Autodesk Inventor part; units mm, degrees
ref_plane "YZ Plane" through (0, 0, 0) normal (1, 0, 0) x (0, 1, 0)
ref_plane "XZ Plane" through (0, 0, 0) normal (0, 1, 0) x (-1, 0, 0)
ref_plane "XY Plane" through (0, 0, 0) normal (0, 0, 1) x (1, 0, 0)
sketch "Esboço1" plane through (0, 0, 0) normal (0, 0, 1) x (1, 0, 0)
  line L0 (-33, -50) -> (-33, 950)
  line L1 (47, -50) -> (47, 950)
  line L2 (-73, -89.8276) -> (47, -89.8276)
  line L3 (47, -9.8276) -> (-73, -9.8276)
  line L4 (-73, -9.8276) -> (-73, -89.8276)
  line L5 (47, -89.8276) -> (47, -9.8276)
  point P0 (0, 0)
  dimension "d0" = 120
  dimension "d1" = 120
  dimension "d2" = 80
extrude "Extrusão1" add sketch "Esboço1" along normal blind 9.52
sketch "Esboço11" plane through (0, 0, 9.52) normal (0, 0, 1) x (1, 0, 0)
  circle A0 centre (-35.5, -47.3276) radius 3
  line L0 (-73, -9.8276) -> (-73, -89.8276)
  point P0 (0, 0)
  dimension "d95" = 6
  dimension "d104" = 37.5
hole "Furo2" at (-35.5, -47.3276, 9.52) direction (0, 0, -1) diameter 4.917 end through all
fillet "Arredondamento3" radius 5 2 edges at (-73, -89.8276, 4.76) (-73, -9.8276, 4.76)
equation "\"d0\" = d1"
properties part number "SUPORTE_GUIA_CORREIA_EIXO_Y"
The listing builds one solid part. Answer for the finished solid, in the listing's coordinates (mm). Round coordinates to 2 decimals unless told otherwise and drop trailing zeros. Loops run counter-clockwise (first coordinate to the right, second up) from the corner with the lowest first, then second, coordinate; pieces in that order, holes last.
1) For a pull along X with two mould halves and no side action, classify faces 1 (the face through (-14, -49, 9.52)), 2 (the face through (-34.56, -49.6, 4.69)), 3 (the face through (47, -50, 5)) as released by +X, released by -X, zero draft, split by the parting line, or undercut.
Outcome:
face 1: zero draft
face 2: undercut
face 3: released by +X
2) Given P1, Ø5, axis at x = -36, y = -54.5, coming from the -Z side; P2, Ø4, axis at x = -35.5, y = -47.33, coming from the -Z side, each flat-ended and moving along its own axis, determine where each tip first touches the part or whether it passes through.
Outcome:
P1: stops at z = 0
P2: passes through
3) A cutting plane is placed at A-A on x = -35.5. Determine the outline of the cut face in (y, z).
Outcome:
outline: (-89.83, 0) - (-49.79, 0) - (-49.79, 9.52) - (-89.83, 9.52) - close; (-44.87, 0) - (-9.83, 0) - (-9.83, 9.52) - (-44.87, 9.52) - close
4) Consider line 1 (Y direction, x = -35.5, z = 7); line 2 (X direction, y = -48, z = 2.75); line 3 (Y direction, x = -36, z = 7.5). Determine where each line is inside the solid, lowest interval first.
Outcome:
line 1: y = -89.83 to -49.79, -44.87 to -9.83
line 2: x = -73 to -37.86, -33.14 to 47
line 3: y = -89.83 to -49.73, -44.92 to -9.83
5) A cutting plane is placed at B-B on y = -46.5. Determine the outline of the cut face in (x, z), plus the area to 3 significant figures.
Outcome:
outline: (-73, 0) - (-37.82, 0) - (-37.82, 9.52) - (-73, 9.52) - close; (-33.18, 0) - (47, 0) - (47, 9.52) - (-33.18, 9.52) - close
area: 1,100 mm2
